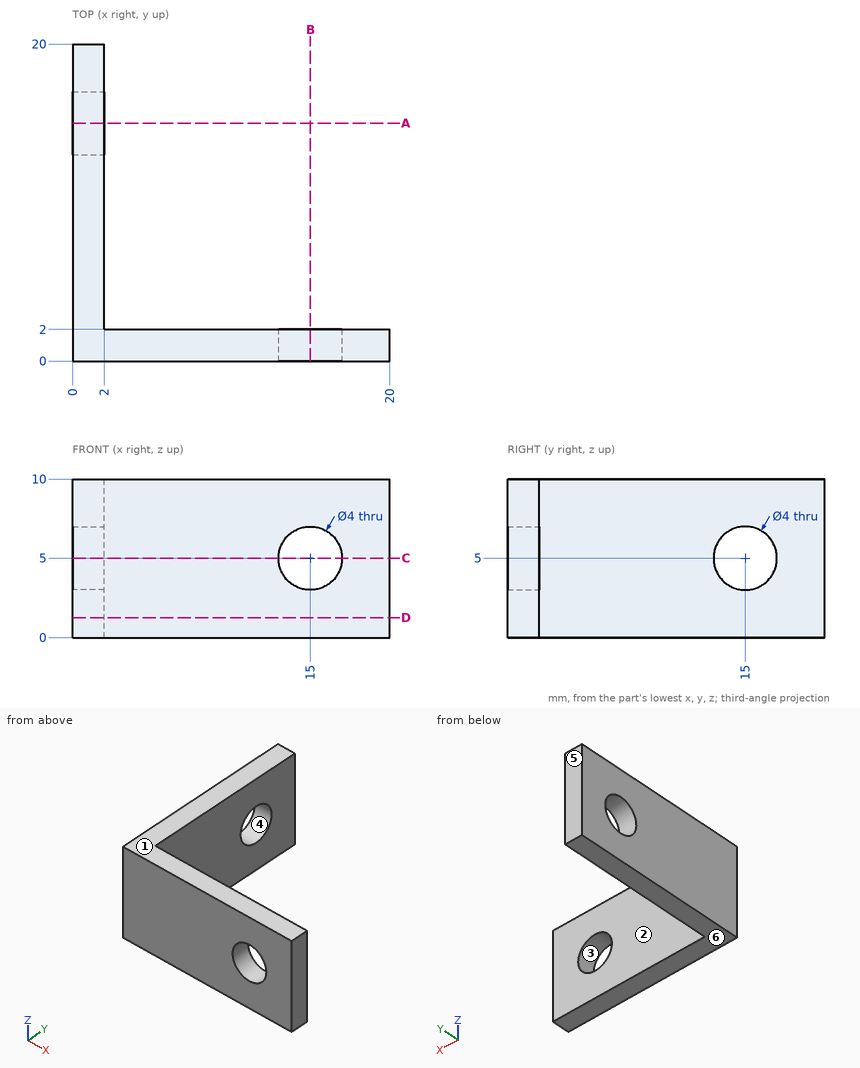
Input: dimensioned drawing with shaded views. Units: mm. Origin: part minimum x, y, z. A direction names the side the tool comes from. Coordinates: 2 decimals unless noted, no trailing zeros. Loops run counter-clockwise (first coordinate to the right, second up) from the corner with the lowest first, then second, coordinate; pieces in that order, holes last. Notation, with made-up numbers: M -34,7.5 L -5,7.5 A18 cw -5,24.5 Z; hole C 83.5,6 d11. An arc over 180 degrees is marked long. Use a Markdown table: item, result. Add a question column.
1) Section D-D, the plane z = 1.25. Return the cut outline in (x, y).
2) Draft query along Z for the marked faces 3, 4, 5 and 6. Return one class per face: +Z half, -Z half, draft (parallel to the pull), parting line (faces both ways), or undercut.
3) Pin query (flat end, axial travel): P1, Ø3.5, axis at x = 15, z = 5, coming from the +Y side; P2, Ø5, axis at y = 14, z = 8.5, coming from the +X side; P3, Ø1.5, axis at x = 8.5, z = 4, coming from the +Y side. Return the tip coordinate at first contact, or that it passes through.
4) Section C-C, the plane z = 5. Return the cut outline in (x, y), plus the area to 3 significant figures.
5) Section A-A, the plane y = 15. Return the cut outline in (x, z).
6) Line query: L1, parallel to Y at x = 1.05, z = 5; L2, parallel to Y at x = 10.75, z = 4; L3, parallel to Z at x = 15, y = 1.3. Output: solid intervals per line, ascending. Write a range as from..to.
7) Set-up query: the marked faces 1 and 2. Return all of +Z, -Z, +X, -X, +Y, -Y with unobstructed straight access to the full face (end or side cutting, diameter ignored); none if empty.
Answer below:
| question | item | result |
|---|---|---|
| 1 | outline | M 0,0 L 20,0 L 20,2 L 2,2 L 2,20 L 0,20 Z |
| 2 | face 3 | undercut |
| 2 | face 4 | undercut |
| 2 | face 5 | draft |
| 2 | face 6 | -Z half |
| 3 | P1 | through |
| 3 | P2 | x = 2 |
| 3 | P3 | y = 2 |
| 4 | outline | M 0,0 L 13,0 L 13,2 L 2,2 L 2,13 L 0,13 Z; M 0,17 L 2,17 L 2,20 L 0,20 Z; M 17,0 L 20,0 L 20,2 L 17,2 Z |
| 4 | area | 60.0 mm2 |
| 5 | outline | M 0,0 L 2,0 L 2,3 L 0,3 Z; M 0,7 L 2,7 L 2,10 L 0,10 Z |
| 6 | L1 | 0..13, 17..20 |
| 6 | L2 | 0..2 |
| 6 | L3 | 0..3, 7..10 |
| 7 | face 1 | +Z, +X, -X, +Y, -Y |
| 7 | face 2 | +Z, -Z, +X, +Y |
